```python
from build123d import *
from build123d import SkipClean  # not in build123d's __all__

# Parameters (mm, degrees)
F1_DEPTH = 63.5
F3_DEPTH = 12.7
F4_DEPTH = 63.501
F6_DEPTH = 12.7
F8_D     = 12.7
F8_DEPTH = 152.4
F8_TIP   = 3.8154649308


# Not quite as in the source:
# - after a boolean that leaves OpenCascade's solid faulty, fix() repairs it


with BuildPart() as f1:
    # F0 (on Front) → F1 (new body)
    with BuildSketch(Plane.XZ):
        Polygon((-29.9473897851, 37.1472596026), (-42.7499328044, 37.1472596026), (-55.5491112173, 37.1472596026), (-55.5491112173, -22.0509488136), (54.1031509638, -22.0509488136), (54.1031509638, 37.1472596026), (41.2416318434, 37.1472596026), (28.4390888242, 37.1472596026), (20.3639920801, 37.1472596026), (-23.0149235576, 37.1472596026), align=None)
    extrude(amount=-F1_DEPTH)

    # F2 (on face) → F3 (join)
    with BuildSketch(Plane.XZ):
        with BuildLine():
            Line((-21.5689614415, 37.1472596026), (-32.8956767917, 37.1472596026))
            ThreePointArc((-32.8956767917, 37.1472596026), (0.1204963773, 4.4575092605), (33.1366695464, 37.1472596026))
            Line((33.1366695464, 37.1472596026), (22.5329399109, 37.1472596026))
            ThreePointArc((22.5329399109, 37.1472596026), (0.4819892347, 13.3748375843), (-21.5689614415, 37.1472596026))
        make_face()
    extrude(amount=F3_DEPTH)

    # F4 (cut, through all): a face of the model
    f4_faces = [f1.faces().sort_by_distance(p)[0] for p in [
        (0.4819892347, 0, 26.9928771395),
    ]]
    extrude(f4_faces, amount=-F4_DEPTH, mode=Mode.SUBTRACT)

    # F5 (on face) → F6 (join)
    with BuildSketch(Plane(origin=(0, 63.5, 0), x_dir=(-1, 0, 0), z_dir=(0, 1, 0))):
        with BuildLine():
            Line((-22.5329399109, 37.1472596026), (-32.1724079549, 37.1472596026))
            ThreePointArc((-32.1724079549, 37.1472596026), (0.7585827261, 1.0699512778), (33.6895734072, 37.1472596026))
            Line((33.6895734072, 37.1472596026), (21.5689614415, 37.1472596026))
            ThreePointArc((21.5689614415, 37.1472596026), (-0.4819892347, 13.3748375843), (-22.5329399109, 37.1472596026))
        make_face()
    with SkipClean():  # cleaning this boolean's faces spoils the solid; the shape is the same uncleaned
        extrude(amount=F6_DEPTH)

    # F8
    with Locations(Plane.XY.offset(37.1472596026)):
        with Locations((-44.2922338843, 31.75), (42.5287522376, 31.75)):
            Hole(F8_D / 2, depth=F8_DEPTH)
            with Locations((0, 0, -(F8_DEPTH + F8_TIP / 2))):  # 118° drill point
                Cone(0, F8_D / 2, F8_TIP, mode=Mode.SUBTRACT)

    add(f1.part.fix(), mode=Mode.REPLACE)


solid = f1.part
```
Work out the finished part from the listing and answer in its coordinate system (mm). A direction names the side the tool comes from. Coordinates: 2 decimals unless noted, no trailing zeros. Loops run counter-clockwise (first coordinate to the right, second up) from the corner with the lowest first, then second, coordinate; pieces in that order, holes last. Notation, with made-up numbers: M 51.25,74 L 93.25,74 A14 ccw 93.25,95 Z; hole C -39.75,43.5 d7. An arc over 180 degrees is marked long. Use CSV: the item, a comma, the result in double quotes. Start each with the question number.
(1) Find section B-B, the plane y = 31.75. Give the vertices of the cut face in (x, z).
(2) Find section C-C, the plane z = -10. Give the vertices of the cut face in (x, y).
(3) For faces 4 (the face through (-8, -12.7, 14)), 5 (the face through (-1, 63.5, -5)), 6 (the face through (-0.601, -6.261, 4.465)), determine the directions among +Z, -Z, +X, -X, +Y, -Y from which every point of the face is accessible in a straight line to the end or side of a thin tool.
(4) Given pin 1 Ø10 at (x, y) = (42.53, 31.75) entering from -Z (1 decimal); pin 2 Ø1 at (x, y) = (-17.5, 47.5) entering from +Z; pin 3 Ø4 at (x, z) = (-1.5, -15) entering from +Y, each flat-ended and moving along its own axis, determine where each tip first touches the part or whether it passes through.
(5) Consider line 1 (X direction, y = 34.5, z = -13); line 2 (Y direction, x = 1.5, z = 1); line 3 (X direction, y = 26, z = 23). Determine where each line is inside the solid, lowest interval first.
(6) Find section D-D, the plane x = -9.5. Give the vertices of the cut face in (y, z), then the cut area to 3 significant figures.
(7) Find section A-A, the plane z = 23.5. Give the vertices of the cut face in (x, y), then the cut area to 3 significant figures.
(8) For a pull along Y with two mould halves and no side action, classify faces 1 (the face through (-55.549, 31, 8)), 2 (the face through (0, 76.2, 11)), 3 (the face through (36.472, 33.657, 7.134)) as +Y half, -Y half, draft (parallel to the pull), parting line (faces both ways), or undercut.
Recorded:
1,outline,"M -55.55,-22.05 L -50.64,-22.05 L -50.64,37.15 L -55.55,37.15 Z; M -37.94,-22.05 L 36.18,-22.05 L 36.18,37.15 L 22.53,37.15 A22.11 cw long -21.57,37.15 L -37.94,37.15 Z; M 48.88,-22.05 L 54.1,-22.05 L 54.1,37.15 L 48.88,37.15 Z"
2,outline,"M -55.55,0 L 54.1,0 L 54.1,63.5 L -55.55,63.5 Z; hole C -44.29,31.75 d12.7; hole C 42.53,31.75 d12.7"
3,face 4,"+Z, -Z, +X, -X, -Y"
3,face 5,"-Z, +Y"
3,face 6,"-Z, -Y"
4,pin 1,"passes through"
4,pin 2,"stops at z = 23.35"
4,pin 3,"stops at y = 63.5"
5,line 1,"x = -55.55 to -50.02, -38.57 to 36.81, 48.25 to 54.1"
5,line 2,"y = 0 to 63.5"
5,line 3,"x = -55.55 to -46.99, -41.6 to -17.77, 18.73 to 39.83, 45.22 to 54.1"
6,outline,"M -12.7,5.89 L 0,5.89 L 0,-22.05 L 63.5,-22.05 L 63.5,2.25 L 76.2,2.25 L 76.2,15.76 L -12.7,15.76 Z"
6,area,"2,700 mm^2"
7,outline,"M -55.55,0 L -29.79,0 L -29.79,-12.7 L -18.1,-12.7 L -18.1,76.2 L -32.07,76.2 L -32.07,63.5 L -55.55,63.5 Z; M 19.06,-12.7 L 30.03,-12.7 L 30.03,0 L 54.1,0 L 54.1,63.5 L 30.55,63.5 L 30.55,76.2 L 19.06,76.2 Z; hole C -44.29,31.75 d12.7; hole C 42.53,31.75 d12.7"
7,area,"4,960 mm^2"
8,face 1,"draft"
8,face 2,"+Y half"
8,face 3,"undercut"
